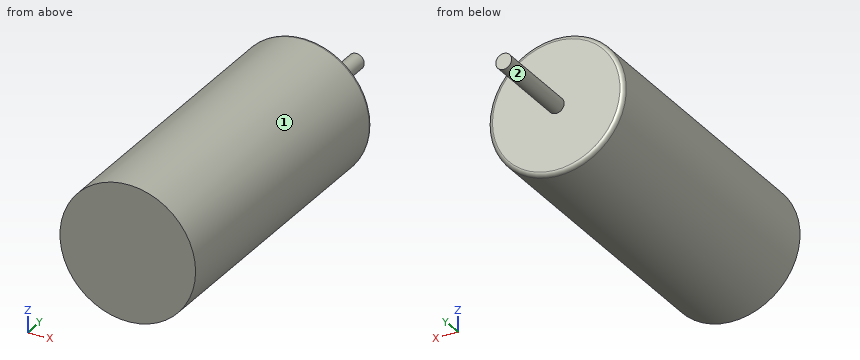
from build123d import *

# Parameters (mm, degrees)
SKETCH1_R           = 4.25
BOSS_EXTRUDE1_DEPTH = 9.652
SKETCH2_R           = 0.4953
BOSS_EXTRUDE2_DEPTH = 5.7658
FILLET1_R           = 0.254


with BuildPart() as part:
    # Sketch1 → Boss-Extrude1 (new body, symmetric)
    with BuildSketch(Plane(origin=(0, 0, 0), x_dir=(1, 0, 0), z_dir=(0, 1, 0))):
        Circle(SKETCH1_R)
    extrude(amount=BOSS_EXTRUDE1_DEPTH, both=True)

    # Sketch2 → Boss-Extrude2 (add)
    with BuildSketch(Plane(origin=(0, 9.652, 0), x_dir=(1, 0, 0), z_dir=(0, 1, 0))):
        Circle(SKETCH2_R)
    extrude(amount=BOSS_EXTRUDE2_DEPTH)

    # Fillet1
    fillet1_edges = [part.edges().sort_by_distance(p)[0] for p in [
        (-4.25, 9.652, 0),
    ]]
    fillet(fillet1_edges, radius=FILLET1_R)


solid = part.part
The model under review builds one solid part; all positions refer to its coordinate system, in mm. Face numbers are marked on the shaded views. A direction names the side the tool comes from. Give positions to 0.01 mm unless a question says otherwise; leave off trailing zeros. Write each loop counter-clockwise with the first axis right and the second up, starting at its lowest first coordinate (ties: lowest second). Pieces come first, ordered by that corner, then holes.
1. Add section A-A, the plane z = 0. Write out the cut boundary in (x, y).
2. Wall thickness on L1, parallel to Y at x = 2, z = 0; L2, parallel to Z at x = -1.5, y = 0.75; L3, parallel to X at y = -6, z = -1: over which ranges is each line inside the solid? List them lowest first.
3. Add section B-B, the plane x = 0. Write out the cut boundary in (y, z), plus the area to 3 significant figures.
4. For P1, Ø5, axis at x = -1, y = 6, coming from the -Z side; P2, Ø3, axis at y = -3.5, z = -2, coming from the -X side; P3, Ø1.5, axis at x = -2, y = 3.5, coming from the +Z side, all flat-tipped, find the tip position at first contact; note any pin that passes through.
5. Add section C-C, the plane y = 1. Write out the cut boundary in (x, z).
6. Tool access review of the marked faces 1 and 2: name each direction out of +Z, -Z, +X, -X, +Y, -Y from which nothing blocks a thin tool from reaching the whole face with its end or side.
7. Add section D-D, the plane y = 11.5. Write out the cut boundary in (x, z), plus the area to 3 significant figures.
Worked answers:
1. outline: (-4.25, -9.65) - (4.25, -9.65) - (4.25, 9.4) arc R0.25 ccw to (4, 9.65) - (0.5, 9.65) - (0.5, 15.42) - (-0.5, 15.42) - (-0.5, 9.65) - (-4, 9.65) arc R0.25 ccw to (-4.25, 9.4) - close
2. L1: y = -9.65 to 9.65
2. L2: z = -3.98 to 3.98
2. L3: x = -4.13 to 4.13
3. outline: (-9.65, -4.25) - (9.4, -4.25) arc R0.25 ccw to (9.65, -4) - (9.65, -0.5) - (15.42, -0.5) - (15.42, 0.5) - (9.65, 0.5) - (9.65, 4) arc R0.25 ccw to (9.4, 4.25) - (-9.65, 4.25) - close
3. area: 170 mm2
4. P1: stops at z = -4.25
4. P2: stops at x = -4.22
4. P3: stops at z = 4.06
5. outline: circle Ø8.5 at (0, 0)
6. face 1: +Y, -Y
6. face 2: +Y
7. outline: circle Ø0.99 at (0, 0)
7. area: 0.771 mm2
